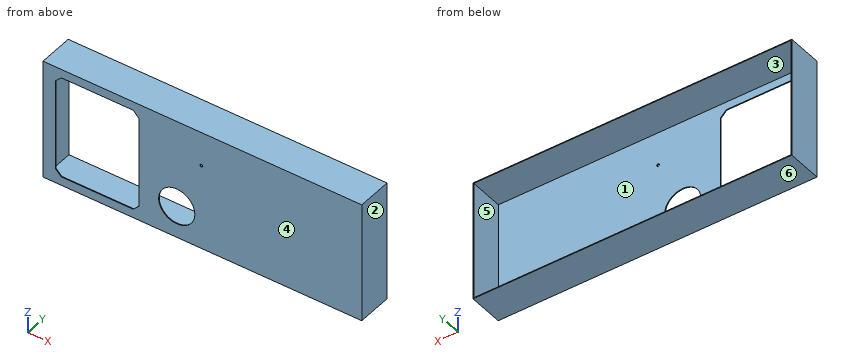
from build123d import *

# Parameters (mm, degrees)
F0_W     = 820
F0_H     = 310
F1_DEPTH = 2
F2_W     = 820
F2_H     = 310
F2_W_2   = 816
F2_H_2   = 306
F3_DEPTH = 88
F5_R     = 46.5
F5_R_2   = 3.5
F6_DEPTH = 90.001


with BuildPart() as f1:
    # F0 (on Front) → F1 (new body)
    with BuildSketch(Plane.XZ):
        with Locations((410, 155)):
            Rectangle(F0_W, F0_H)
    extrude(amount=F1_DEPTH)

    # F2 (on face) → F3 (join)
    with BuildSketch(Plane(origin=(0, 0, 0), x_dir=(-1, 0, 0), z_dir=(0, 1, 0))):
        with Locations((-410, 155)):
            Rectangle(F2_W, F2_H)
        with Locations((-410, 155)):
            Rectangle(F2_W_2, F2_H_2, mode=Mode.SUBTRACT)
    extrude(amount=F3_DEPTH)

    # F5 (on face) → F6 (cut, through all)
    with BuildSketch(Plane.XZ.offset(2)):
        Polygon((47.000004, 287.499992), (32.000004, 272.499992), (32.000004, 37.499992), (47.000004, 22.499992), (232.000004, 22.499992), (247.000004, 37.499992), (247.000004, 272.499992), (232.000004, 287.499992), align=None)
        with Locations((344.000004, 82.749992)):
            Circle(F5_R)
        with Locations((407.500004, 221.499992)):
            Circle(F5_R_2)
    extrude(amount=-F6_DEPTH, mode=Mode.SUBTRACT)


solid = f1.part
Could you check a few things on this model? Use its own coordinates, in mm. Face numbers are marked on the shaded views. A direction names the side the tool comes from. Give positions to 0.01 mm unless a question says otherwise; leave off trailing zeros. Order: outer loops, then holes, each group sorted by start corner. A loop starts at its lowest first (then second) coordinate and runs counter-clockwise, first axis right, second up. Notation, with made-up numbers: M -12,21 L -8,21 A31 ccw -8,53 Z; hole C 37,78 d1. An arc over 180 degrees is marked long. One line per question, with ' | ' between items.
1. I want a section at C-C (x = 703). List the corners of the cut face in (y, z) for me, and give its area (3 significant figures).
Results:
outline: M -2,0 L 88,0 L 88,2 L 0,2 L 0,308 L 88,308 L 88,310 L -2,310 Z | area: 972 mm²
2. I want a section at A-A (z = 186). List the corners of the cut face in (x, y) for me.
Results:
outline: M 0,-2 L 32,-2 L 32,0 L 2,0 L 2,88 L 0,88 Z; M 247,-2 L 820,-2 L 820,88 L 818,88 L 818,0 L 247,0 Z
3. If I drill on line 1 (Z direction, x = 485, y = 56); line 2 (X direction, y = 60.5, z = 38.5); line 3 (Y direction, x = 308, z = 175), over which ranges is the centre line in solid material (lowest first)?
Results:
line 1: 0 to 2, 308 to 310 | line 2: 0 to 2, 818 to 820 | line 3: -2 to 0
4. I want a section at B-B (y = 66). List the corners of the cut face in (x, z) for me, and give its area (3 significant figures).
Results:
outline: M 0,0 L 820,0 L 820,310 L 0,310 Z; hole M 2,2 L 818,2 L 818,308 L 2,308 Z | area: 4,500 mm²
5. I'm going to push flat-ended pins straight in: pin 1 (0.6 mm diameter, centred on y = -1, z = 167.5, fed in from -X); pin 2 (6 mm diameter, centred on x = 701, z = 230.5, fed in from +Y). Where does each tip first touch, or does it pass through?
Results:
pin 1: x = 0 | pin 2: y = 0
6. We'd pull the mould along X, two halves only. Please class the marked faces 1, 2, 3 and 4: +X half, -X half, draft (parallel to the pull), parting line (faces both ways), or undercut.
Results:
face 1: undercut | face 2: +X half | face 3: undercut | face 4: draft
7. For the marked faces 5 and 6, which set-ups out of +Z, -Z, +X, -X, +Y, -Y let a thin tool reach every point of the face, with its end or its side?
Results:
face 5: +Y | face 6: -Z, +X, -X, +Y, -Y
8. I want a section at D-D (z = 93.5). List the corners of the cut face in (x, y) for me, and give its area (3 significant figures).
Results:
outline: M 0,-2 L 32,-2 L 32,0 L 2,0 L 2,88 L 0,88 Z; M 247,-2 L 298.76,-2 L 298.76,0 L 247,0 Z; M 389.24,-2 L 820,-2 L 820,88 L 818,88 L 818,0 L 389.24,0 Z | area: 1,380 mm²
